For this review, take the finished solid that the model builds, in its own axes (mm). A direction names the side the tool comes from. Give positions to 0.01 mm unless a question says otherwise; leave off trailing zeros. Order: outer loops, then holes, each group sorted by start corner. A loop starts at its lowest first (then second) coordinate and runs counter-clockwise, first axis right, second up. Notation, with made-up numbers: (48, -1) - (59, -1) arc R29 ccw to (59, 38) - close; hole circle Ø11 at (17, 62). An arc over 180 degrees is marked (long way). Put each result on its own line as item: value. Start each with the question number.
Autodesk Inventor part; units mm, degrees
ref_plane "Work Plane2" through (0, 32, 0) normal (0, 1, 0) x (1, 0, 0)
ref_plane "Work Plane3" through (-66, 32, -4) normal (0, 0, -1) x (-1, 0, 0)
ref_plane "YZ Plane" through (0, 0, 0) normal (1, 0, 0) x (0, 1, 0)
sketch "Sketch1" plane through (0, 0, 0) normal (0, 1, 0) x (-1, 0, 0)
  line L0 (0, 0) -> (70, 0)
  line L1 (70, 0) -> (70, -100)
  line L2 (70, -100) -> (0, -100)
  line L3 (0, -100) -> (0, 0)
  circle A0 centre (35, -100) radius 35
  point P0 (0, -100)
  dimension "d0" = 70
  dimension "d1" = 100
extrude "Extrusion1" add sketch "Sketch1" along normal blind 35
chamfer "Chamfer1" distance 5 angle 45 3 edges at (0, 0, -50) (-35, 0, -135) (-70, 0, -50)
shell "Shell1" thickness 4 removed faces 1 at (-23.3333, 35, -33.3333)
sketch "Sketch2" plane through (-70, 0, 0) normal (0, 0, 1) x (1, 0, 0)
  line L0 (35, 44.7542) -> (35, -30.4775) construction
  line L1 (75.874, 17.5) -> (-5.874, 17.5) construction
  line L2 (0, 35) -> (70, 35)
  line L3 (70, 0) -> (70, 35)
  line L4 (0, 0) -> (0, 35)
  line L5 (0, 0) -> (70, 0)
  line L6 (58, 23) -> (12, 23)
  line L7 (12, 23) -> (12, 12)
  line L8 (12, 12) -> (58, 12)
  line L9 (58, 12) -> (58, 23)
  circle A0 centre (10, 27.5) radius 2.5
  circle A1 centre (60, 7.5) radius 2.5
  circle A2 centre (10, 7.5) radius 2.5
  circle A3 centre (60, 27.5) radius 2.5
  point P0 (35, 17.5)
  point P1 (35, 35)
  point P2 (70, 17.5)
  dimension "d7" = 12
  dimension "d8" = 5
  dimension "d9" = 50
  dimension "d10" = 20
extrude "Extrusion2" cut sketch "Sketch2" against normal blind 50 contours L9 L8 L7 L6 | A0 | A1 | A2 | A3
ref_plane "Work Plane2" through (0, 32, 0) normal (0, 1, 0) x (1, 0, 0)
sketch "Sketch4" plane through (0, 32, 0) normal (0, 1, 0) x (1, 0, 0)
  line L0 (-66, 4) -> (-66, 100)
  arc A0 (-4, 100) -> (-66, 100) centre (-35, 100) ccw
  line L1 (-4, 100) -> (-4, 4)
  line L2 (-4, 4) -> (-66, 4)
  point P0 (0, 0)
ref_plane "Work Plane3" through (-66, 32, -4) normal (0, 0, -1) x (-1, 0, 0)
sketch "Sketch5" plane through (-66, 32, -4) normal (0, 0, -1) x (-1, 0, 0)
  line L0 (0, 1) -> (1, 0)
  line L1 (1, 0) -> (0, -1)
  line L2 (0, -1) -> (0, 1)
  line L3 (2.655, 0) -> (0.8949, 0) construction
  point P0 (-66, -32)
  point P1 (0, 0)
  point P2 (0, 0)
  point P3 (0, 0)
  dimension "d29" = 1
  dimension "d30" = 45
sweep "Sweep1" cut profiles "Sketch5" path "Sketch4"
sketch "Sketch6" plane through (-35, 4, -100) normal (0, 1, 0) x (1, 0, 0)
  circle A0 centre (-21, 0) radius 2.15
  circle A1 centre (21, 0) radius 2.15
  line L0 (0, -2.8251) -> (0, 10.2985) construction
  arc A2 (31, 0) -> (-31, 0) centre (0, 0) ccw
  line L1 (3, -25) -> (-3, -25) construction
  line L2 (3, -22) -> (-3, -22)
  line L3 (-3, -28) -> (3, -28)
  arc A3 (3, -28) -> (3, -22) centre (3, -25) ccw
  arc A4 (-3, -22) -> (-3, -28) centre (-3, -25) ccw
  point P0 (35, -100)
  point P1 (0, 31)
  point P2 (0, -25)
  dimension "d33" = 4.3
  dimension "d34" = 42
  dimension "d37" = 6
  dimension "d38" = 6
  dimension "d39" = 25
extrude "Extrusion5" cut sketch "Sketch6" against normal blind 50
sketch "Sketch7" plane through (-35, 4, -100) normal (0, 1, 0) x (1, 0, 0)
  line L0 (-23.0785, 3.6) -> (-18.9215, 3.6)
  line L1 (-18.9215, 3.6) -> (-16.8431, 0)
  line L2 (-16.8431, 0) -> (-18.9215, -3.6)
  line L3 (-18.9215, -3.6) -> (-23.0785, -3.6)
  line L4 (-23.0785, -3.6) -> (-25.1569, 0)
  line L5 (-25.1569, 0) -> (-23.0785, 3.6)
  circle A0 centre (-21, 0) radius 2.15
  circle A1 centre (21, 0) radius 2.15
  line L6 (23.0785, 3.6) -> (25.1569, 0)
  line L7 (25.1569, 0) -> (23.0785, -3.6)
  line L8 (23.0785, -3.6) -> (18.9215, -3.6)
  line L9 (18.9215, -3.6) -> (16.8431, 0)
  line L10 (16.8431, 0) -> (18.9215, 3.6)
  line L11 (18.9215, 3.6) -> (23.0785, 3.6)
  point P0 (35, -100)
  point P1 (-21, -3.6)
  dimension "d40" = 7.2
extrude "Extrusion6" cut sketch "Sketch7" against normal blind 2
fillet "Fillet1" radius 4 4 edges at (-58, 12, -2) (-58, 23, -2) (-12, 23, -2) (-12, 12, -2)
equation "\"d11\" = d9"
equation "\"d35\" = d9"
properties part number "SCARA arm"
1. Tool access review of faces 1 (the face through (-56.47, 1.01, -97.9)), 2 (the face through (-13.203, 21.859, -2.028)), 3 (the face through (-35.682, 18.658, -130.993)): name each direction out of +Z, -Z, +X, -X, +Y, -Y from which nothing blocks a thin tool from reaching the whole face with its end or side.
2. Add section D-D, the plane z = -37.5. Give the boundary of the cut face in (x, y), then the cut area to 3 significant figures.
3. Add section B-B, the plane x = -35. Give the boundary of the cut face in (y, z), then the cut area to 3 significant figures.
4. The part is to be moulded in two halves that separate along Y. For faces 4 (the face through (-3, 2, -49)), 5 (the face through (-64.653, 5.31, -52.672)), 6 (the face through (-4, 19, -53)), 7 (the face through (-13.141, 13.203, -2.028)), say which applies: released by +Y, released by -Y, zero draft, split by the parting line, or undercut.
5. Wall thickness on line 1 (X direction, y = 1, z = -100); line 2 (Y direction, x = -60, z = -1.95); line 3 (X direction, y = 23.5, z = -37.5): over which ranges is each line inside the solid? List them lowest first. Write a range as from..to.
6. Add section A-A, the plane z = -75. Give the boundary of the cut face in (x, y).
7. Clearance check with flat-ended pins moving along their axes: pin 1 (10 mm diameter, centred on x = -26.5, z = -29.5, fed in from +Y); pin 2 (12 mm diameter, centred on x = -27, y = 12, fed in from -Z); pin 3 (1.5 mm diameter, centred on x = -52, y = 11, fed in from -Z). State where each tip first meets the part, or that it passes through.
8. Add section C-C, the plane y = 27.5. Give the boundary of the cut face in (x, z).
Found:
1. face 1: +Y, -Y
1. face 2: +Z
1. face 3: +Y
2. outline: (-70, 5) - (-65, 0) - (-5, 0) - (0, 5) - (0, 35) - (-4, 35) - (-4, 33) - (-3, 32) - (-4, 31) - (-4, 6.66) - (-6.66, 4) - (-63.34, 4) - (-66, 6.66) - (-66, 31) - (-67, 32) - (-66, 33) - (-66, 35) - (-70, 35) - close
2. area: 508 mm^2
3. outline: (0, -130) - (5, -135) - (35, -135) - (35, -131) - (33, -131) - (32, -132) - (31, -131) - (6.66, -131) - (4, -128.34) - (4, -78) - (0, -78) - close; (0, -72) - (4, -72) - (4, -4) - (12, -4) - (12, 0) - (0, 0) - close; (23, -4) - (31, -4) - (32, -3) - (33, -4) - (35, -4) - (35, 0) - (23, 0) - close
3. area: 709 mm^2
4. face 4: released by -Y
4. face 5: released by +Y
4. face 6: zero draft
4. face 7: undercut
5. line 1: x = -66..-58.15, -53.85..-16.15, -11.85..-4
5. line 2: y = 0..5, 10..25, 30..35
5. line 3: x = -70..-66, -4..0
6. outline: (-70, 5) - (-65, 0) - (-41, 0) - (-41, 4) - (-63.34, 4) - (-66, 6.66) - (-66, 31) - (-67, 32) - (-66, 33) - (-66, 35) - (-70, 35) - close; (-29, 0) - (-5, 0) - (0, 5) - (0, 35) - (-4, 35) - (-4, 33) - (-3, 32) - (-4, 31) - (-4, 6.66) - (-6.66, 4) - (-29, 4) - close
7. pin 1: stops at y = 4
7. pin 2: stops at z = -134.94
7. pin 3: stops at z = -131
8. outline: (-70, -100) arc R35 ccw to (0, -100) - (0, 0) - (-7.5, 0) - (-7.5, -4) - (-4, -4) - (-4, -100) arc R31 cw to (-66, -100) - (-66, -4) - (-62.5, -4) - (-62.5, 0) - (-70, 0) - close; (-57.5, -4) - (-12.5, -4) - (-12.5, 0) - (-57.5, 0) - close
